Verification items for the finished model (mm, model axes). Round coordinates to 2 decimals unless told otherwise and drop trailing zeros. Write each loop counter-clockwise with the first axis right and the second up, starting at its lowest first coordinate (ties: lowest second). Pieces come first, ordered by that corner, then holes. Notation, with made-up numbers: (-37, 54.5) -> (21, 54.5) arc R17 ccw to (21, 62.5) -> close; hole circle Ø8 at (86, -3). An arc over 180 degrees is marked (long way). Answer as a JSON object with one key per item and string values. Group by question number.
(1) Draft check along X on faces 1 (the face through (24, 2, 0)), 2 (the face through (3.65, 1.57, -25.01)), 3 (the face through (0, 2, -19)). Enter one of: released by +X, released by -X, zero draft, split by the parting line, or undercut.
(2) Sectioned sample at A-A on x = 23.5. Record the cut outline in (y, z) (3 decimals).
(3) Sectioned sample at B-B on z = -26. Record the cut outline in (x, y) (3 decimals), and give its area (3 significant figures).
(4) Gauge pin test, flat end, axial feed: pin 1 Ø2 at (x, z) = (37.79, -22.54) entering from -Y. Record the tip position at first contact, or that the pin passes through.
(5) Sectioned sample at C-C on y = 1.85. Count the separate pieces of the cut face and the enclosed holes in it, and give its area (3 significant figures).
(6) Scan lines: L1, parallel to X at y = 2.45, z = -14.5; L2, parallel to X at y = 2.65, z = -6; L3, parallel to X at y = 2.15, z = -27.5. Record each from-to range of solid material in increasing order. Write a range as from..to.
```python
from build123d import *

# Parameters (mm, degrees)
SKETCH1_W           = 49.53
SKETCH1_H           = 38.1
BOSS_EXTRUDE1_DEPTH = 3.175
SKETCH4_R           = 1.190625
SKETCH4_R_2         = 6.35
SKETCH4_R_3         = 1.5875
CUT_EXTRUDE2_DEPTH  = 63.569253831


with BuildPart() as part:
    # Sketch1 → Boss-Extrude1 (new body)
    with BuildSketch(Plane(origin=(0, 0, 0), x_dir=(1, 0, 0), z_dir=(0, 1, 0))):
        with Locations((24.765, 19.05)):
            Rectangle(SKETCH1_W, SKETCH1_H)
    extrude(amount=BOSS_EXTRUDE1_DEPTH)

    # Sketch4 → Cut-Extrude2 (cut, through all)
    with BuildSketch(Plane.XZ):
        with Locations(Location((21.274204011, -6.022172011, 0), (0, 0, 270))):
            Circle(SKETCH4_R)
        with Locations(Location((37.792827989, -22.540795989, 0), (0, 0, 270))):
            Circle(SKETCH4_R)
        with Locations(Location((15.227967999, -28.587032001, 0), (0, 0, 270))):
            Circle(SKETCH4_R)
        with Locations(Location((24.765, -25.7048, 0), (0, 0, 270))):
            Circle(SKETCH4_R_2)
        with Locations(Location((3.175, -23.495, 0), (0, 0, 270))):
            Circle(SKETCH4_R_3)
        with Locations(Location((3.175, -14.605, 0), (0, 0, 90))):
            Circle(SKETCH4_R_3)
        with Locations(Location((46.355, -14.605, 0), (0, 0, 270))):
            Circle(SKETCH4_R_3)
        with Locations(Location((46.355, -23.495, 0), (0, 0, 90))):
            Circle(SKETCH4_R_3)
    extrude(amount=-CUT_EXTRUDE2_DEPTH, mode=Mode.SUBTRACT)


solid = part.part
```
Computed values:
{
 "1": {"face 1": "zero draft", "face 2": "undercut", "face 3": "released by -X"},
 "2": {"outline": "(0, -38.1) -> (3.175, -38.1) -> (3.175, -31.928) -> (0, -31.928) -> close; (0, -19.482) -> (3.175, -19.482) -> (3.175, 0) -> (0, 0) -> close"},
 "3": {"outline": "(0, 0) -> (18.422, 0) -> (18.422, 3.175) -> (0, 3.175) -> close; (31.108, 0) -> (49.53, 0) -> (49.53, 3.175) -> (31.108, 3.175) -> close", "area": "117 mm2"},
 "4": {"pin 1": "through"},
 "5": {"separate pieces": "1", "enclosed holes": "8", "area": "1,720 mm2"},
 "6": {"L1": "0..1.59, 4.76..44.77, 47.94..49.53", "L2": "0..20.08, 22.46..49.53", "L3": "0..14.74, 15.71..18.67, 30.86..49.53"}
}
